```python
from build123d import *

# Parameters (mm, degrees)
F2_W     = 7.161952
F2_H     = 3
F3_DEPTH = 6.2


with BuildPart() as f1:
    # F0 (on Front) → F1 (revolve)
    with BuildSketch(Plane.XZ):
        Polygon((0, 8.75), (0, 0), (4.55, 0), (4.55, 1.35), (2.45, 1.35), (2.45, 8.75), (1.85, 9.35), (0.6, 9.35), align=None)
    revolve(axis=Axis((0, 0, 11.047808), (0, 0, 1)))

    # F2 (on face) → F3 (cut)
    with BuildSketch(Plane.XY.offset(9.35)):
        with Locations((0.21525, 3)):
            Rectangle(F2_W, F2_H)
        with Locations((0.21525, -3)):
            Rectangle(F2_W, F2_H)
    extrude(amount=-F3_DEPTH, mode=Mode.SUBTRACT)


solid = f1.part
```
Read the model definition and answer for the solid it produces. Units are mm, in the model's axes. A direction names the side the tool comes from. Give positions to 0.01 mm unless a question says otherwise; leave off trailing zeros. Order: outer loops, then holes, each group sorted by start corner. A loop starts at its lowest first (then second) coordinate and runs counter-clockwise, first axis right, second up.
(1) Find section B-B (z = 4.25). Give the vertices of the cut face in (x, y).
(2) Find section D-D (z = 1.75). Give the vertices of the cut face in (x, y).
(3) Find section A-A (y = 1.75). Give the vertices of the cut face in (x, z).
(4) For a pull along X with two mould halves and no side action, classify faces 1 (the flat face through (0, 1.5, 6)), 2 (the conical face through (2, 0, 9.2)), 3 (the conical face through (-0.129, -0.099, 8.912)) as released by +X, released by -X, zero draft, split by the parting line, or undercut.
(5) Find section C-C (x = 3.75). Give the vertices of the cut face in (y, z).
(6) Straight lines are drawn through the part: L1, parallel to Z at x = -3.75, y = 0.25; L2, parallel to Y at x = 1.5, z = 7.75; L3, parallel to Y at x = 2, z = 0.5. For each, find the intervals that lie inside material, in ascending order.
(7) Given pin 1 (0.8 mm diameter, centred on x = -0.5, y = -2, fed in from +Z); pin 2 (3 mm diameter, centred on x = -0.5, z = 5, fed in from +Y); pin 3 (3 mm diameter, centred on x = 2.5, y = 3.5, fed in from +Z), each flat-ended and moving along its own axis, determine where each tip first touches the part or whether it passes through.
(8) For faces 4 (the cylindrical face through (2.263, -0.938, 4.28)), 5 (the flat face through (0, 1, 9.35)), 6 (the flat face through (0, -1.5, 6)), 7 (the flat face through (0, 2, 3.15)), determine the directions among +Z, -Z, +X, -X, +Y, -Y from which every point of the face is accessible in a straight line to the end or side of a thin tool.
Result sheet:
1. outline: (-1.94, -1.5) - (1.94, -1.5) arc R2.45 ccw to (1.94, 1.5) - (-1.94, 1.5) arc R2.45 ccw to start
2. outline: circle Ø4.9 at (0, 0)
3. outline: (-4.2, 0) - (4.2, 0) - (4.2, 1.35) - (1.71, 1.35) - (1.71, 3.15) - (-1.71, 3.15) - (-1.71, 1.35) - (-4.2, 1.35) - close
4. face 1: zero draft
4. face 2: released by +X
4. face 3: undercut
5. outline: (-2.58, 0) - (2.58, 0) - (2.58, 1.35) - (-2.58, 1.35) - close
6. L1: z = 0 to 1.35
6. L2: y = -1.5 to 1.5
6. L3: y = -4.09 to 4.09
7. pin 1: stops at z = 3.15
7. pin 2: stops at y = 1.5
7. pin 3: stops at z = 1.35
8. face 4: +Z
8. face 5: +Z, +X, -X, +Y, -Y
8. face 6: +Z, +X, -X, -Y
8. face 7: +Z, +X, -X, +Y
